```python
from build123d import *

# Parameters (mm, degrees)
CYLINDER001_R               = 12.8
CYLINDER001_DEPTH           = 2.3
CYLINDER001_ROLL_ANGLE      = 89.8666565593
CYLINDER001_PITCH_ANGLE     = -0.0557418137
CYLINDER001_PLACEMENT_ANGLE = -45.3729530145
SKETCH022_W                 = 35
SKETCH022_H                 = 45.6
PAD010_DEPTH                = 32
SKETCH023_W                 = 27
SKETCH023_H                 = 50
POCKET008_DEPTH             = 28
SKETCH024_W                 = 31
SKETCH024_H                 = 5
POCKET009_DEPTH             = 29
PAD009_DEPTH                = 14
POCKET007_DEPTH             = 6
SKETCH028_W                 = 4
SKETCH028_H                 = 28
POCKET011_DEPTH             = 28
PAD012_DEPTH                = 5
SKETCH030_W                 = 3.15
SKETCH030_H                 = 36
POCKET012_DEPTH             = 7
CUT002_PLACEMENT_ANGLE      = 90
CYLINDER_R                  = 12.8
CYLINDER_DEPTH              = 2.3
CYLINDER_ROLL_ANGLE         = 89.8666565593
CYLINDER_PITCH_ANGLE        = -0.0557418137
CYLINDER_PLACEMENT_ANGLE    = -45.3729530145
SKETCH017_W                 = 35
SKETCH017_H                 = 45.6
PAD008_DEPTH                = 32
SKETCH018_W                 = 27
SKETCH018_H                 = 50
POCKET005_DEPTH             = 28
SKETCH019_W                 = 31
SKETCH019_H                 = 5
POCKET006_DEPTH             = 29
PAD_DEPTH                   = 14
POCKET_DEPTH                = 6
PAD011_DEPTH                = 5
SKETCH027_W                 = 35
SKETCH027_H                 = 3.15
POCKET010_DEPTH             = 7


with BuildPart() as obj1:
    # Cylinder001 → Cylinder001 (new body)
    with BuildSketch(Plane.XY):
        Circle(CYLINDER001_R)
    extrude(amount=CYLINDER001_DEPTH)


with BuildPart() as obj1_1:
    # Cylinder001 roll: moved
    add(obj1.part.rotate(Axis((0, 0, 0), (1, 0, 0)), CYLINDER001_ROLL_ANGLE))


with BuildPart() as obj1_2:
    # Cylinder001 pitch: moved
    add(obj1_1.part.rotate(Axis((0, 0, 0), (0, 1, 0)), CYLINDER001_PITCH_ANGLE))


with BuildPart() as obj1_3:
    # Cylinder001 placement: moved
    add(obj1_2.part.moved(Location((-38.25, -74, 18))).rotate(Axis((-38.25, -74, 18), (0, 0, 1)), CYLINDER001_PLACEMENT_ANGLE))


with BuildPart() as base02:
    # Sketch022 → Pad010 (new body)
    with BuildSketch(Plane.XY):
        Rectangle(SKETCH022_W, SKETCH022_H)
    extrude(amount=PAD010_DEPTH)

    # Sketch023 (on Face6 of Pad010) → Pocket008 (cut)
    with BuildSketch(Plane.XY.offset(32)):
        Rectangle(SKETCH023_W, SKETCH023_H)
    extrude(amount=-POCKET008_DEPTH, mode=Mode.SUBTRACT)

    # Sketch024 (on Face4 of Pocket008) → Pocket009 (cut)
    with BuildSketch(Plane.XY.offset(32)):
        with Locations((0, 17.3)):
            Rectangle(SKETCH024_W, SKETCH024_H)
    extrude(amount=-POCKET009_DEPTH, mode=Mode.SUBTRACT)

    # Sketch021 (on Face17 of Pocket009) → Pad009 (join)
    with BuildSketch(Plane.XY.offset(4)):
        Polygon((-12.73, -0.3126406871), (8.4832034356, -21.5258441227), (12.7258441227, -17.2832034356), (-8.4873593129, 3.93), align=None)
    extrude(amount=PAD009_DEPTH)

    # Sketch025 (on Face19 of Pad009) → Pocket007 (cut)
    with BuildSketch(Plane(origin=(-6.5213203436, -6.5213203436, 0), x_dir=(0.7071067812, -0.7071067812, 0), z_dir=(-0.7071067812, -0.7071067812, 0))):
        with BuildLine():
            ThreePointArc((-5.7803989746, 18), (6.2196010254, 6), (18.2196010254, 18))
            Line((-5.7803989746, 18), (18.2196010254, 18))
        make_face()
    extrude(amount=-POCKET007_DEPTH, mode=Mode.SUBTRACT)

    # Sketch028 (on Face6 of Pocket007) → Pocket011 (cut)
    with BuildSketch(Plane.XY.offset(32)):
        with Locations((15.5, -4.8)):
            Rectangle(SKETCH028_W, SKETCH028_H)
    extrude(amount=-POCKET011_DEPTH, mode=Mode.SUBTRACT)

    # Sketch029 (on Face4 of Pocket011) → Pad012 (join)
    with BuildSketch(Plane.YZ.offset(17.5)):
        Polygon((-22.8, 0), (-22.8, 10), (-18.8, 10), (-18.8, 4), (9.2, 4), (9.2, 10), (13.2, 10), (13.2, 0), align=None)
    extrude(amount=PAD012_DEPTH)

    # Sketch030 (on Face30 of Pad012) → Pocket012 (cut)
    with BuildSketch(Plane.XY.offset(10)):
        with Locations((19.075, -4.8)):
            Rectangle(SKETCH030_W, SKETCH030_H)
    extrude(amount=-POCKET012_DEPTH, mode=Mode.SUBTRACT)


with BuildPart() as base02_1:
    # Body007 placement: moved
    add(base02.part.moved(Location((-39, -66, 0))))

    # Cut002: cut obj1
    add(obj1_3.part, mode=Mode.SUBTRACT)


with BuildPart() as base02_2:
    # Cut002 placement: moved
    add(base02_1.part.moved(Location((67, -44.3, 0))).rotate(Axis((67, -44.3, 0), (0, 0, -1)), CUT002_PLACEMENT_ANGLE))


with BuildPart() as obj2:
    # Cylinder → Cylinder (new body)
    with BuildSketch(Plane.XY):
        Circle(CYLINDER_R)
    extrude(amount=CYLINDER_DEPTH)


with BuildPart() as obj2_1:
    # Cylinder roll: moved
    add(obj2.part.rotate(Axis((0, 0, 0), (1, 0, 0)), CYLINDER_ROLL_ANGLE))


with BuildPart() as obj2_2:
    # Cylinder pitch: moved
    add(obj2_1.part.rotate(Axis((0, 0, 0), (0, 1, 0)), CYLINDER_PITCH_ANGLE))


with BuildPart() as obj2_3:
    # Cylinder placement: moved
    add(obj2_2.part.moved(Location((-38.25, -8, 18))).rotate(Axis((-38.25, -8, 18), (0, 0, 1)), CYLINDER_PLACEMENT_ANGLE))


with BuildPart() as obj3:
    # Sketch017 → Pad008 (new body)
    with BuildSketch(Plane.XY):
        Rectangle(SKETCH017_W, SKETCH017_H)
    extrude(amount=PAD008_DEPTH)

    # Sketch018 (on Face6 of Pad008) → Pocket005 (cut)
    with BuildSketch(Plane.XY.offset(32)):
        Rectangle(SKETCH018_W, SKETCH018_H)
    extrude(amount=-POCKET005_DEPTH, mode=Mode.SUBTRACT)

    # Sketch019 (on Face4 of Pocket005) → Pocket006 (cut)
    with BuildSketch(Plane.XY.offset(32)):
        with Locations((0, 17.3)):
            Rectangle(SKETCH019_W, SKETCH019_H)
    extrude(amount=-POCKET006_DEPTH, mode=Mode.SUBTRACT)

    # Sketch (on Face17 of Pocket006) → Pad (join)
    with BuildSketch(Plane.XY.offset(4)):
        Polygon((-12.73, -0.3126406871), (8.4832034356, -21.5258441227), (12.7258441227, -17.2832034356), (-8.4873593129, 3.93), align=None)
    extrude(amount=PAD_DEPTH)

    # Sketch020 (on Face19 of Pad) → Pocket (cut)
    with BuildSketch(Plane(origin=(-6.5213203436, -6.5213203436, 0), x_dir=(0.7071067812, -0.7071067812, 0), z_dir=(-0.7071067812, -0.7071067812, 0))):
        with BuildLine():
            ThreePointArc((-5.7803989746, 18), (6.2196010254, 6), (18.2196010254, 18))
            Line((-5.7803989746, 18), (18.2196010254, 18))
        make_face()
    extrude(amount=-POCKET_DEPTH, mode=Mode.SUBTRACT)

    # Sketch026 (on Face10 of Pocket) → Pad011 (join)
    with BuildSketch(Plane.XZ.offset(22.8)):
        Polygon((-17.5, 0), (17.5, 0), (17.5, 10), (13.5, 10), (13.5, 4), (-13.5, 4), (-13.5, 10), (-17.5, 10), align=None)
    extrude(amount=PAD011_DEPTH)

    # Sketch027 (on Face22 of Pad011) → Pocket010 (cut)
    with BuildSketch(Plane.XY.offset(10)):
        with Locations((0, -24.375)):
            Rectangle(SKETCH027_W, SKETCH027_H)
    extrude(amount=-POCKET010_DEPTH, mode=Mode.SUBTRACT)


with BuildPart() as obj3_1:
    # Body006 placement: moved
    add(obj3.part.moved(Location((-39, 0, 0))))

    # Cut001: cut obj2
    add(obj2_3.part, mode=Mode.SUBTRACT)

    # Fusion: union Base02
    add(base02_2.part)


solid = obj3_1.part
```
Verification items for the finished model (mm, model axes). A direction names the side the tool comes from. Coordinates: 2 decimals unless noted, no trailing zeros. Write each loop counter-clockwise with the first axis right and the second up, starting at its lowest first coordinate (ties: lowest second). Pieces come first, ordered by that corner, then holes. Notation, with made-up numbers: M 19,24 L 78,24 A10 ccw 78,35 Z; hole C 35,22 d7. An arc over 180 degrees is marked long. One line per item, written item: value.
Item 1: Access from +Z, -Z, +X, -X, +Y, -Y to the whole of each face (thin tool, end or side, straight path). Record for faces 1 (the flat face through (2, 4, 18)), 2 (the flat face through (1, 12.2, 16)), 3 (the flat face through (22, -18.8, 18)).
Check sheet entries:
face 1: +Z, +X, -Y
face 2: +Z, -Z, +X, +Y
face 3: +Z, +X
Item 2: Scan lines: line 1 along X through (y, z) = (10, 28.5); line 2 along X through (y, z) = (1, 14); line 3 along X through (y, z) = (19, 23). Record each from-to range of solid material in increasing order.
Check sheet entries:
line 1: x = -56.5 to -52.5, -25.5 to 15.8, 20.8 to 23.8
line 2: x = -56.5 to -52.5, -50.42 to -45.2, -25.5 to -21.5, 1.9 to 2.74
line 3: x = -56.5 to -54.5, -23.5 to -21.5
Item 3: Mould release check, pull along Y, two halves, no side actions. Record for faces 4 (the flat face through (-36.73, -6.83, 4.68)), 5 (the flat face through (-25.5, 21, 18)), 6 (the cylindrical face through (-9, -4, 6)): pulls with the +Y half, pulls with the -Y half, needs draft (parallel to the pull), parting line crosses it, or undercut.
Check sheet entries:
face 4: pulls with the +Y half
face 5: needs draft
face 6: undercut
Item 4: Section check B-B, the plane x = 13. Record the boundary of the cut face in (y, z).
Check sheet entries:
outline: M -27.8,0 L 12.2,0 L 12.2,32 L 8.2,32 L 8.2,4 L -18.8,4 L -18.8,32 L -22.8,32 L -22.8,3 L -25.95,3 L -25.95,10 L -27.8,10 Z
Item 5: Section check A-A, the plane z = 21. State how many separate pieces and enclosed holes the cut face has, plus the area to 3 significant figures.
Check sheet entries:
separate pieces: 3
enclosed holes: 0
area: 575 mm^2
Item 6: Gauge pin test, flat ends, axial feed: pin 1 Ø1.9 at (x, y) = (-18, -14.5) entering from +Z; pin 2 Ø4 at (x, y) = (1.5, 16) entering from +Z; pin 3 Ø1.5 at (x, z) = (22.5, 20) entering from +Y; pin 4 Ø3.5 at (x, y) = (-37.5, 21.5) entering from +Z. Record the tip position at first contact, or that the pin passes through.
Check sheet entries:
pin 1: stops at z = 18
pin 2: passes through
pin 3: stops at y = 12.2
pin 4: stops at z = 4
